```python
from build123d import *

# Parameters (mm, degrees)
F1_DEPTH = 7
F2_R     = 1


with BuildPart() as f1:
    # F0 (on Top) → F1 (new body)
    with BuildSketch(Plane.XY):
        with BuildLine():
            Line((0, 3.967148), (0, 6.770925))
            Line((0, 6.770925), (2, 6.770925))
            Line((2, 6.770925), (2, 16.770925))
            Line((2, 16.770925), (0.187763, 16.770925))
            Line((0.187763, 16.770925), (-1.624474, 11.770925))
            Line((-1.624474, 11.770925), (-1.624474, 7.852102))
            ThreePointArc((-1.624474, 7.852102), (-1.976897, 7.090101), (-2.785764, 6.865195))
            ThreePointArc((-2.785764, 6.865195), (-4.908971, 7.563736), (-6.715642, 8.879756))
            Line((-6.715642, 8.879756), (-8.695541, 6.899857))
            ThreePointArc((-8.695541, 6.899857), (-5.461971, 4.736554), (-1.647563, 3.970952))
            Line((-1.647563, 3.970952), (0, 3.967148))
        make_face()
        with BuildLine():
            ThreePointArc((-6.715642, 8.879756), (-8.695541, 8.879756), (-8.695541, 6.899857))
            Line((-8.695541, 6.899857), (-6.715642, 8.879756))
        make_face()
    extrude(amount=F1_DEPTH)

    # F2
    f2_edges = [f1.edges().sort_by_distance(p)[0] for p in [
        (0, 6.770925, 3.5),
    ]]
    fillet(f2_edges, radius=F2_R)


solid = f1.part
```
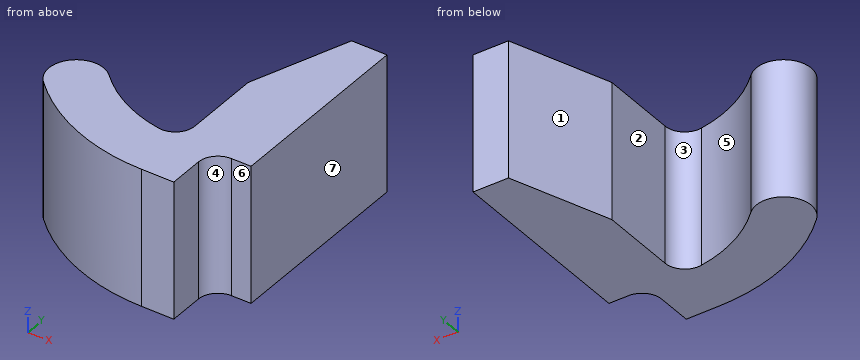
The listing builds one solid part. Answer for the finished solid, in the listing's coordinates (mm). Face numbers are marked on the shaded views. A direction names the side the tool comes from. Coordinates: 2 decimals unless noted, no trailing zeros. Loops run counter-clockwise (first coordinate to the right, second up) from the corner with the lowest first, then second, coordinate; pieces in that order, holes last. Notation, with made-up numbers: (-40, 27.5) - (16, 27.5) arc R32 cw to (16, 61.5) - close; hole circle Ø10 at (53, 38). An arc over 180 degrees is marked (long way). Use a Markdown table: item, result. Add a question column.
1) Find the intervals of material crossed by line 1 (X direction, y = 11.75, z = 3.25); line 2 (X direction, y = 8.5, z = 1.5); line 3 (Y direction, x = -7.25, z = 2.5), in increasing order.
2) The part is cut by section B-B, the plane y = 10.5. Give the vertices of the cut face in (x, z), and give its area (3 significant figures).
3) For the marked faces 5, 6 and 7, determine the directions among +Z, -Z, +X, -X, +Y, -Y from which every point of the face is accessible in a straight line to the end or side of a thin tool.
4) The part is cut by section C-C, the plane x = -3.5. Give the vertices of the cut face in (y, z).
5) The mould has two halves that part along X. Classify the marked faces 1, 2, 3 and 4: released by +X, released by -X, zero draft, split by the parting line, or undercut.
6) Given pin 1 (2 mm diameter, centred on y = 9, z = 4.5, fed in from -X); pin 2 (4 mm diameter, centred on x = -4, z = 1, fed in from +Y); pin 3 (1 mm diameter, centred on x = -5, y = 6, fed in from -Z); pin 4 (0.9 mm diameter, centred on y = 4.5, z = 4.5, fed in from +X), each flat-ended and moving along its own axis, determine where each tip first touches the part or whether it passes through.
7) The part is cut by section A-A, the plane z = 1.5. Give the vertices of the cut face in (x, y).
Here are the results:
| question | item | result |
|---|---|---|
| 1 | line 1 | x = -1.62 to 2 |
| 1 | line 2 | x = -8.97 to -6.31, -1.62 to 2 |
| 1 | line 3 | y = 5.7 to 9.21 |
| 2 | outline | (-1.62, 0) - (2, 0) - (2, 7) - (-1.62, 7) - close |
| 2 | area | 25.4 mm^2 |
| 3 | face 5 | +Z, -Z, +Y |
| 3 | face 6 | +Z, -Z, +X, -Y |
| 3 | face 7 | +Z, -Z, +X, +Y, -Y |
| 4 | outline | (4.15, 0) - (7.02, 0) - (7.02, 7) - (4.15, 7) - close |
| 5 | face 1 | released by -X |
| 5 | face 2 | undercut |
| 5 | face 3 | undercut |
| 5 | face 4 | released by +X |
| 6 | pin 1 | stops at x = -9.1 |
| 6 | pin 2 | stops at y = 8.25 |
| 6 | pin 3 | stops at z = 0 |
| 6 | pin 4 | stops at x = 0 |
| 7 | outline | (-8.7, 6.9) arc R10 ccw to (-1.65, 3.97) - (0, 3.97) - (0, 5.77) arc R1 cw to (1, 6.77) - (2, 6.77) - (2, 16.77) - (0.19, 16.77) - (-1.62, 11.77) - (-1.62, 7.85) arc R1 cw to (-2.79, 6.87) arc R7.2 cw to (-6.72, 8.88) arc R1.4 ccw to start |
